```python
from build123d import *

# Parameters (mm, degrees)
F1_DEPTH = 8
F6_R     = 4
F7_SIZE  = 2


with BuildPart() as f1:
    # F0 (on Top) → F1 (new body)
    with BuildSketch(Plane.XY):
        Polygon((5.732233047, -5.732233047), (0, 0), (-5.732233047, -5.732233047), (-12.4497474683, -12.4497474683), (-10.3284271247, -14.5710678119), (0, -4.2426406871), (10.3284271247, -14.5710678119), (12.4497474683, -12.4497474683), align=None)
        Polygon((-5.732233047, -5.732233047), (0, 0), (5.732233047, -5.732233047), (5.732233047, -2.732233047), (0, 3), (-5.732233047, -2.732233047), align=None)
    extrude(amount=F1_DEPTH)

    # F3 (on face) → F4 section 0
    with BuildSketch(Plane(origin=(0, 0, 0), x_dir=(-0.7071067812, 0.7071067812, 0), z_dir=(0.7071067812, 0.7071067812, 0))):
        with BuildLine():
            add(Edge.make_bspline(
                [(-10.0066017178, 4), (-10.0066017178, 7.204293994), (-13.1566017178, 5.602146997), (-16.3066017178, 4), (-13.1566017178, 2.397853003), (-10.0066017178, 0.795706006), (-10.0066017178, 4)],
                knots=[0, 0, 0, 2.0943951024, 2.0943951024, 4.1887902048, 4.1887902048, 6.2831853072, 6.2831853072, 6.2831853072], degree=2, weights=[1, 0.5, 1, 0.5, 1, 0.5, 1]))
        make_face()
    # F2 (on face) → F4 section 1
    with BuildSketch(Plane(origin=(-2.1213203436, -2.1213203436, 0), x_dir=(0.7071067812, -0.7071067812, 0), z_dir=(-0.7071067812, -0.7071067812, 0))):
        with BuildLine():
            add(Edge.make_bspline(
                [(11.5066017178, 4), (11.5066017178, 0.795706006), (14.6566017178, 2.397853003), (17.8066017178, 4), (14.6566017178, 5.602146997), (11.5066017178, 7.204293994), (11.5066017178, 4)],
                knots=[0, 0, 0, 2.0943951024, 2.0943951024, 4.1887902048, 4.1887902048, 6.2831853072, 6.2831853072, 6.2831853072], degree=2, weights=[1, 0.5, 1, 0.5, 1, 0.5, 1]))
        make_face()
    f4 = loft(mode=Mode.SUBTRACT)

    # F5: F4 across plane
    add(f4.mirror(Plane.YZ), mode=Mode.SUBTRACT)

    # F6
    f6_edges = [f1.edges().sort_by_distance(p)[0] for p in [
        (0, -4.242641, 4),
        (0, 3, 4),
    ]]
    fillet(f6_edges, radius=F6_R)

    # F7
    f7_edges = [f1.edges().sort_by_distance(p)[0] for p in [
        (11.389087, -13.510408, 8),
        (11.389087, -13.510408, 0),
        (-11.389087, -13.510408, 8),
        (-11.389087, -13.510408, 0),
    ]]
    chamfer(f7_edges, length=F7_SIZE)


solid = f1.part
```
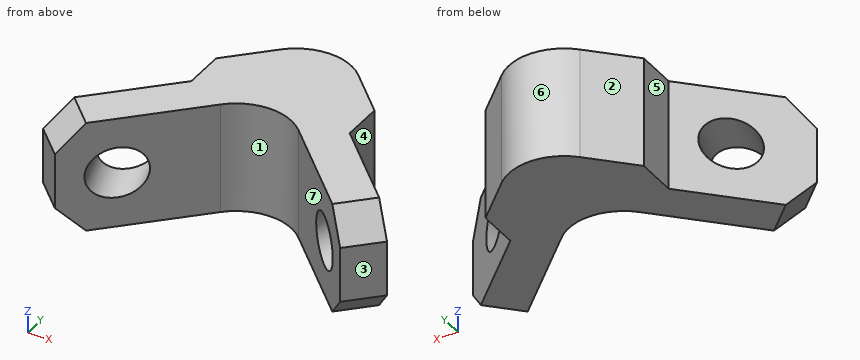
The model under review builds one solid part; all positions refer to its coordinate system, in mm. Face numbers are marked on the shaded views. A direction names the side the tool comes from. Coordinates: 2 decimals unless noted, no trailing zeros. Write each loop counter-clockwise with the first axis right and the second up, starting at its lowest first coordinate (ties: lowest second). Pieces come first, ordered by that corner, then holes. Notation, with made-up numbers: (43, 18) -> (47, 18) arc R25 ccw to (47, 31) -> close; hole circle Ø3 at (-23, -26). An arc over 180 degrees is marked (long way). One line per item, written item: value. Start each with the question number.
Q1. Add section C-C, the plane z = 2.5. Count the separate pieces of the cut face and the enclosed holes in it, then the cut area to 3 significant figures.
Q2. Add section A-A, the plane y = -1.25. Give the boundary of the cut face in (x, z).
Q3. To check wall thickness, follow probe 1 along X at (y, z) = (-2.75, 2); probe 2 along Z at (x, y) = (-6.75, -8.75); probe 3 along X at (y, z) = (-7, 5.5). State the ranges of each line that lie inside material, in increasing order.
Q4. For the marked faces 4, 5, 6 and 7, list the 3-axis set-ups (+Z, -Z, +X, -X, +Y, -Y) from which the entire face can be reached by the end or side of a thin tool; tool diameter is ignored.
Q5. The part is to be moulded in two halves that separate along X. For the marked faces 1, 2 and 3, say which applies: +X half, -X half, draft (parallel to the pull), parting line (faces both ways), or undercut.
Q6. Clearance check with flat-ended pins moving along their axes: P1, Ø2.5, axis at y = -5, z = 4.5, coming from the -X side; P2, Ø2.5, axis at y = -4, z = 5.5, coming from the +X side; P3, Ø2, axis at x = -8.5, z = 4, coming from the -Y side. State where each tip first meets the part, or that it passes through.
Q7. Add section D-D, the plane x = 5. Give the boundary of the cut face in (y, z), then the cut area to 3 significant figures.
Q8. Add section B-B, the plane z = 1.25. Give the boundary of the cut face in (x, y), then the cut area to 3 significant figures.
Response:
1. separate pieces: 3
1. enclosed holes: 0
1. area: 116 mm²
2. outline: (-4.25, 0) -> (4.25, 0) -> (4.25, 8) -> (-4.25, 8) -> close
3. probe 1: -5.73 to 5.73
3. probe 2: 0 to 3.13, 4.87 to 8
3. probe 3: -7 to -2.76, 2.76 to 7
4. face 4: +Z, -Z, +X, +Y
4. face 5: +Z, -Z, -X, +Y
4. face 6: +Z, -Z, +Y
4. face 7: +Z, -Z, -Y
5. face 1: undercut
5. face 2: -X half
5. face 3: +X half
6. P1: x = -6.25
6. P2: x = 5.73
6. P3: y = -13.74
7. outline: (-9.24, 0) -> (-2, 0) -> (-2, 8) -> (-9.24, 8) -> close
7. area: 57.9 mm²
8. outline: (-11.92, -11.92) -> (-9.8, -14.04) -> (-2.83, -7.07) arc R4 cw to (2.83, -7.07) -> (9.8, -14.04) -> (11.92, -11.92) -> (5.73, -5.73) -> (5.73, -2.73) -> (2.83, 0.17) arc R4 ccw to (-2.83, 0.17) -> (-5.73, -2.73) -> (-5.73, -5.73) -> close
8. area: 127 mm²
